Can you work these out from the model? Positions are in its coordinate system, mm. A direction names the side the tool comes from. Coordinates: 2 decimals unless noted, no trailing zeros. Order: outer loops, then holes, each group sorted by start corner. A loop starts at its lowest first (then second) coordinate and runs counter-clockwise, first axis right, second up. Notation, with made-up numbers: (18, 9) -> (39, 9) arc R23 ccw to (39, 31) -> close; hole circle Ø3 at (80.5, 88). An arc over 180 degrees is marked (long way). Answer in a Markdown table with one row per item.
```python
from build123d import *

# Parameters (mm, degrees)
SKETCH1_W                                    = 101.6
SKETCH1_H                                    = 83.312
SOLID_EXTRUDE_DEPTH                          = 234.95
BOTTOM_SLIDE_WAY_CUT_EXTRUDE_DEPTH           = 270.193149697
THROAT_CASTING_CUT_EXTRUDE_DEPTH             = 270.193149697
SHOULDERS_SCREW_HOLE_CUT_EXTRUDE_REACH       = 271.193
SKETCH4_R                                    = 7.9375
CBORE_START                                  = -38.1
CBORE_FOR_M6_PAN_HEAD_MACHINE_SCREW1_OUT_R   = 3.3
CBORE_FOR_M6_PAN_HEAD_MACHINE_SCREW1_DEPTH   = 38.1
CBORE_START_2                                = -4.6
CBORE_FOR_M6_PAN_HEAD_MACHINE_SCREW1_2_O_R   = 6.5
CBORE_FOR_M6_PAN_HEAD_MACHINE_SCREW1_2_O_R_2 = 3.3
CBORE_FOR_M6_PAN_HEAD_MACHINE_SCREW1_2_DEPTH = 4.6
SKETCH7_W                                    = 38.1
SKETCH7_H                                    = 10.922
STATIONARY_JAW_TRIM_CUT_EXTRUDE1_DEPTH       = 270.193149697
F_1_4_20_TAPPED_HOLE1_D                      = 5.1054
F_1_4_20_TAPPED_HOLE1_DEPTH                  = 14.986
F_1_4_20_TAPPED_HOLE1_TIP                    = 1.533816902
F_10_32_TAPPED_HOLE1_D                       = 4.0386
F_10_32_TAPPED_HOLE1_DEPTH                   = 11.938
F_10_32_TAPPED_HOLE1_TIP                     = 1.213317848


# Read off the part's stored shape, not the designer's step: CBORE for M6 Pan Head Machine Screw1
with BuildPart() as part:
    # Sketch1 → Solid extrude (new body)
    with BuildSketch(Plane.XY):
        with Locations((50.8, 41.656)):
            Rectangle(SKETCH1_W, SKETCH1_H)
    extrude(amount=-SOLID_EXTRUDE_DEPTH)

    # Sketch2 → Bottom slide way cut extrude (cut, through all)
    with BuildSketch(Plane.XY):
        with BuildLine():
            Line((19.431, 0), (19.763794004, 6.35008787))
            ThreePointArc((19.763794004, 6.35008787), (20.84487401, 8.695131686), (23.243283382, 9.652))
            Line((23.243283382, 9.652), (25.781, 9.652))
            Line((25.781, 9.652), (26.326795038, 11.151559542))
            ThreePointArc((26.326795038, 11.151559542), (26.849188972, 11.832356572), (27.667598166, 12.0904))
            Line((27.667598166, 12.0904), (31.75, 12.0904))
            Line((31.75, 12.0904), (31.75, 38.1))
            Line((31.75, 38.1), (69.85, 38.1))
            Line((69.85, 38.1), (69.85, 12.0904))
            Line((69.85, 12.0904), (73.932401834, 12.0904))
            ThreePointArc((73.932401834, 12.0904), (74.750811028, 11.832356572), (75.273204962, 11.151559542))
            Line((75.273204962, 11.151559542), (75.819, 9.652))
            Line((75.819, 9.652), (78.356716618, 9.652))
            ThreePointArc((78.356716618, 9.652), (80.75512599, 8.695131686), (81.836205996, 6.35008787))
            Line((81.836205996, 6.35008787), (82.169, 0))
            Line((82.169, 0), (19.431, 0))
        make_face()
    extrude(amount=-BOTTOM_SLIDE_WAY_CUT_EXTRUDE_DEPTH, mode=Mode.SUBTRACT)

    # Sketch3 → Throat/casting cut extrude (cut, through all)
    with BuildSketch(Plane(origin=(101.6, 0, 0), x_dir=(0, 0, -1), z_dir=(1, 0, 0))):
        with BuildLine():
            Line((0, 74.58075), (19.05, 74.58075))
            ThreePointArc((19.05, 74.58075), (23.540128061, 76.440621939), (25.4, 80.93075))
            Line((25.4, 80.93075), (25.4, 83.312))
            Line((25.4, 83.312), (0, 83.312))
            Line((0, 83.312), (0, 74.58075))
        make_face()
        with BuildLine():
            Line((38.1, 83.312), (38.1, 38.1))
            Line((38.1, 38.1), (187.198, 38.1))
            ThreePointArc((187.198, 38.1), (193.548, 31.75), (199.898, 38.1))
            Line((199.898, 38.1), (199.898, 83.312))
            Line((199.898, 83.312), (38.1, 83.312))
        make_face()
    extrude(amount=-THROAT_CASTING_CUT_EXTRUDE_DEPTH, mode=Mode.SUBTRACT)

    # Sketch4 → Shoulders/screw hole cut extrude (cut, up to next)
    with BuildSketch(Plane(origin=(0, 0, -234.95), x_dir=(-1, 0, 0), z_dir=(0, 0, -1)), mode=Mode.PRIVATE) as shoulders_screw_hole_cut_extrude_sk1:
        with Locations((-50.8, 59.436)):
            Circle(SKETCH4_R)
    shoulders_screw_hole_cut_extrude_tool1 = extrude(shoulders_screw_hole_cut_extrude_sk1.sketch, amount=-SHOULDERS_SCREW_HOLE_CUT_EXTRUDE_REACH, mode=Mode.PRIVATE) & part.part
    # Sketch4 → Shoulders/screw hole cut extrude (cut, up to next)
    with BuildSketch(Plane(origin=(0, 0, -234.95), x_dir=(-1, 0, 0), z_dir=(0, 0, -1)), mode=Mode.PRIVATE) as shoulders_screw_hole_cut_extrude_sk2:
        with BuildLine():
            Line((-2.794, 57.15), (0, 57.15))
            Line((0, 57.15), (0, 83.312))
            Line((0, 83.312), (-28.956, 83.312))
            ThreePointArc((-28.956, 83.312), (-21.293327609, 64.812672391), (-2.794, 57.15))
        make_face()
    shoulders_screw_hole_cut_extrude_tool2 = extrude(shoulders_screw_hole_cut_extrude_sk2.sketch, amount=-SHOULDERS_SCREW_HOLE_CUT_EXTRUDE_REACH, mode=Mode.PRIVATE) & part.part
    # Sketch4 → Shoulders/screw hole cut extrude (cut, up to next)
    with BuildSketch(Plane(origin=(0, 0, -234.95), x_dir=(-1, 0, 0), z_dir=(0, 0, -1)), mode=Mode.PRIVATE) as shoulders_screw_hole_cut_extrude_sk3:
        with BuildLine():
            Line((-101.6, 57.15), (-101.6, 83.312))
            Line((-101.6, 83.312), (-72.644, 83.312))
            ThreePointArc((-72.644, 83.312), (-80.306672391, 64.812672391), (-98.806, 57.15))
            Line((-98.806, 57.15), (-101.6, 57.15))
        make_face()
    shoulders_screw_hole_cut_extrude_tool3 = extrude(shoulders_screw_hole_cut_extrude_sk3.sketch, amount=-SHOULDERS_SCREW_HOLE_CUT_EXTRUDE_REACH, mode=Mode.PRIVATE) & part.part
    add(shoulders_screw_hole_cut_extrude_tool1.solids().sort_by_distance((50.8, 59.436, -234.95))[0], mode=Mode.SUBTRACT)
    add(shoulders_screw_hole_cut_extrude_tool2.solids().sort_by_distance((12.401182, 71.971794, -234.95))[0], mode=Mode.SUBTRACT)
    add(shoulders_screw_hole_cut_extrude_tool3.solids().sort_by_distance((89.198818, 71.971794, -234.95))[0], mode=Mode.SUBTRACT)

    # CBORE for M6 Pan Head Machine Screw1 out → CBORE for M6 Pan Head Machine Screw1 (cut)
    with BuildSketch(Plane.XY.offset(CBORE_START)):
        with Locations((80.187245779, 53.586240129)):
            Circle(CBORE_FOR_M6_PAN_HEAD_MACHINE_SCREW1_OUT_R)
        with Locations((20.004838326, 53.586240129)):
            Circle(CBORE_FOR_M6_PAN_HEAD_MACHINE_SCREW1_OUT_R)
    extrude(amount=CBORE_FOR_M6_PAN_HEAD_MACHINE_SCREW1_DEPTH, mode=Mode.SUBTRACT)

    # CBORE for M6 Pan Head Machine Screw1 2 o → CBORE for M6 Pan Head Machine Screw1 2 (cut)
    # profile 1 of 2: a face of its own
    with BuildSketch(Plane.XY.offset(CBORE_START_2)):
        with Locations((80.187245779, 53.586240129)):
            Circle(CBORE_FOR_M6_PAN_HEAD_MACHINE_SCREW1_2_O_R)
        with Locations((80.187245779, 53.586240129)):
            Circle(CBORE_FOR_M6_PAN_HEAD_MACHINE_SCREW1_2_O_R_2, mode=Mode.SUBTRACT)
    # profile 2 of 2: a face of its own
    with BuildSketch(Plane.XY.offset(CBORE_START_2)):
        with Locations((20.004838326, 53.586240129)):
            Circle(CBORE_FOR_M6_PAN_HEAD_MACHINE_SCREW1_2_O_R)
        with Locations((20.004838326, 53.586240129)):
            Circle(CBORE_FOR_M6_PAN_HEAD_MACHINE_SCREW1_2_O_R_2, mode=Mode.SUBTRACT)
    extrude(amount=CBORE_FOR_M6_PAN_HEAD_MACHINE_SCREW1_2_DEPTH, mode=Mode.SUBTRACT)

    # Sketch7 → Stationary jaw trim Cut-Extrude1 (cut, through all)
    with BuildSketch(Plane(origin=(101.6, 0, 0), x_dir=(0, 0, -1), z_dir=(1, 0, 0))):
        with Locations((19.05, 77.851)):
            Rectangle(SKETCH7_W, SKETCH7_H)
    extrude(amount=-STATIONARY_JAW_TRIM_CUT_EXTRUDE1_DEPTH, mode=Mode.SUBTRACT)

    # 1/4-20 Tapped Hole1
    with Locations(Plane(origin=(50.8, 72.39, 0), x_dir=(-1, 0, 0), z_dir=(0, 1, 0))):
        with Locations((19.05, -19.05), (-19.05, -19.05)):
            Hole(F_1_4_20_TAPPED_HOLE1_D / 2, depth=F_1_4_20_TAPPED_HOLE1_DEPTH)
            with Locations((0, 0, -(F_1_4_20_TAPPED_HOLE1_DEPTH + F_1_4_20_TAPPED_HOLE1_TIP / 2))):  # 118° drill point
                Cone(0, F_1_4_20_TAPPED_HOLE1_D / 2, F_1_4_20_TAPPED_HOLE1_TIP, mode=Mode.SUBTRACT)

    # #10-32 Tapped Hole1
    with Locations(Plane(origin=(0, 0, 0), x_dir=(-1, 0, 0), z_dir=(0, -1, 0))):
        with Locations((-9.7155, 88.9), (-9.7155, 44.45), (-9.7155, 133.35), (-91.8845, 44.45), (-91.8845, 88.9), (-91.8845, 133.35)):
            Hole(F_10_32_TAPPED_HOLE1_D / 2, depth=F_10_32_TAPPED_HOLE1_DEPTH)
            with Locations((0, 0, -(F_10_32_TAPPED_HOLE1_DEPTH + F_10_32_TAPPED_HOLE1_TIP / 2))):  # 118° drill point
                Cone(0, F_10_32_TAPPED_HOLE1_D / 2, F_10_32_TAPPED_HOLE1_TIP, mode=Mode.SUBTRACT)


solid = part.part
```
(1) Suppose I cut it at C-C (y = 22). Please give me the cut outline in (x, z).
Response values:
| item | result |
|---|---|
| outline | (0, -234.95) -> (31.75, -234.95) -> (31.75, 0) -> (0, 0) -> close; (69.85, -234.95) -> (101.6, -234.95) -> (101.6, 0) -> (69.85, 0) -> close |
(2) On a 3-axis mill with a long thin cutter (end or side, diameter ignored), from which of +Z, -Z, +X, -X, +Y, -Y can I reach the whole of each face in a straight line? I mean faces 3 (the cylindrical face through (21.5, 65.02, -217.67)), 4 (the flat face through (72, 12.09, -116)), 5 (the flat face through (52, 72.39, -19)), 6 (the cylindrical face through (83.68, 59.07, -2.33)), 7 (the cylindrical face through (89.867, 6.053, -44.539)). Say none if no direction works.
Response values:
| item | result |
|---|---|
| face 3 | -Z, -X, +Y |
| face 4 | +Z, -Z, -Y |
| face 5 | +Z, +X, -X, +Y |
| face 6 | +Z |
| face 7 | -Y |
(3) Suppose I cut it at D-D (x = 50.8). Please give me the cut outline in (y, z), and give its area (3 significant figures).
Response values:
| item | result |
|---|---|
| outline | (38.1, -234.95) -> (51.5, -234.95) -> (51.5, -199.9) -> (38.1, -199.9) -> close; (38.1, -38.1) -> (72.39, -38.1) -> (72.39, 0) -> (38.1, 0) -> close; (67.37, -234.95) -> (83.31, -234.95) -> (83.31, -199.9) -> (67.37, -199.9) -> close |
| area | 2,330 mm2 |
(4) I need wall thicknesses on line 1 (X direction, y = 6.5, z = -44.45); line 2 (Z direction, x = 69.85, y = 65.75); line 3 (X direction, y = 66.5, z = -19.05). Which ranges of each line are inside material? Lowest first, please. Write a range as [from, to].
Response values:
| item | result |
|---|---|
| line 1 | [0, 7.7], [11.73, 19.77], [81.83, 89.87], [93.9, 101.6] |
| line 2 | [-234.95, -199.9], [-38.1, -21.6], [-16.5, 0] |
| line 3 | [0, 29.2], [34.3, 67.3], [72.4, 101.6] |
(5) Suppose I cut it at A-A (z = -177.5). Please give me the cut outline in (x, y), and give its area (3 significant figures).
Response values:
| item | result |
|---|---|
| outline | (0, 0) -> (19.43, 0) -> (19.76, 6.35) arc R3.48 cw to (23.24, 9.65) -> (25.78, 9.65) -> (26.33, 11.15) arc R1.43 cw to (27.67, 12.09) -> (31.75, 12.09) -> (31.75, 38.1) -> (0, 38.1) -> close; (69.85, 12.09) -> (73.93, 12.09) arc R1.43 cw to (75.27, 11.15) -> (75.82, 9.65) -> (78.36, 9.65) arc R3.48 cw to (81.84, 6.35) -> (82.17, 0) -> (101.6, 0) -> (101.6, 38.1) -> (69.85, 38.1) -> close |
| area | 2,160 mm2 |
(6) Suppose I cut it at B-B (x = 63). Please give me the cut outline in (y, z), and give its area (3 significant figures).
Response values:
| item | result |
|---|---|
| outline | (38.1, -234.95) -> (83.31, -234.95) -> (83.31, -199.9) -> (38.1, -199.9) -> close; (38.1, -38.1) -> (72.39, -38.1) -> (72.39, 0) -> (38.1, 0) -> close |
| area | 2,890 mm2 |
(7) Will these pins go through, and if not, where does the flat tip stop? pin 1 Ø1.3 at (x, z) = (77, -93) entering from -Y; pin 2 Ø4.5 at (x, z) = (91.88, -44.45) entering from +Y; pin 3 Ø2 at (x, z) = (1.5, -214) entering from +Y.
Response values:
| item | result |
|---|---|
| pin 1 | y = 9.65 |
| pin 2 | y = 38.1 |
| pin 3 | y = 57.15 |
(8) We'd pull the mould along Z, two halves only. Please class faces 1 (the cylindrical face through (9.45, 6.05, -90.9)), 2 (the cylindrical face through (80.1, 65.02, -217.67)): +Z half, -Z half, draft (parallel to the pull), parting line (faces both ways), or undercut.
Response values:
| item | result |
|---|---|
| face 1 | undercut |
| face 2 | draft |
